Read the model definition and answer for the solid it produces. Units are mm, in the model's axes. A direction names the side the tool comes from. Coordinates: 2 decimals unless noted, no trailing zeros. Loops run counter-clockwise (first coordinate to the right, second up) from the corner with the lowest first, then second, coordinate; pieces in that order, holes last. Notation, with made-up numbers: (29.25, -32.5) -> (82.25, -32.5) arc R15 cw to (82.25, -9.5) -> close; hole circle Ø10 at (35.25, -6.75). An arc over 180 degrees is marked (long way). Answer as CSV lines item,"result".
```python
from build123d import *

# Parameters (mm, degrees)
F2_SIZE2 = 1
F2_SIZE  = 1


with BuildPart() as f1:
    # F0 (on Front) → F1 (revolve)
    with BuildSketch(Plane.XZ):
        Polygon((4, 35), (0, 35), (0, -35), (4, -35), (4, -33), (3, -33), (3, -32), (4, -32), (4, 32), (3, 32), (3, 33), (4, 33), align=None)
    revolve(axis=Axis((0, 0, 0), (0, 0, -1)))

    # F2
    f2_edges = [f1.edges().sort_by_distance(p)[0] for p in [
        (-4, 0, 35),
        (-4, 0, -35),
    ]]
    chamfer(f2_edges, length=F2_SIZE, length2=F2_SIZE2)


solid = f1.part
```
Q1. For faces 1 (the face through (-1, -3, 33)), 2 (the face through (-0.867, 3.905, 0.448)), determine the directions among +Z, -Z, +X, -X, +Y, -Y from which every point of the face is accessible in a straight line to the end or side of a thin tool.
Results:
face 1,"none"
face 2,"+Z, -Z"
Q2. Find the intervals of material crossed by probe 1 along Z at (x, y) = (-2.5, -2.75); probe 2 along Z at (x, y) = (-3, -2); probe 3 along X at (y, z) = (0.25, -10), in increasing order. Write a range as [from, to].
Results:
probe 1,"z = [-34.28, -33], [-32, 32], [33, 34.28]"
probe 2,"z = [-34.39, -33], [-32, 32], [33, 34.39]"
probe 3,"x = [-3.99, 3.99]"
Q3. A cutting plane is placed at A-A, the plane z = 1. Write down the section's boundary in (x, y), and give its area (3 significant figures).
Results:
outline,"circle Ø8 at (0, 0)"
area,"50.3 mm²"
Q4. For a pull along Z with two mould halves and no side action, classify faces 3 (the face through (1, -3, 32)), 4 (the face through (-0.867, 3.905, 33.507)), 5 (the face through (0, 0, 35)) as pulls with the +Z half, pulls with the -Z half, needs draft (parallel to the pull), parting line crosses it, or undercut.
Results:
face 3,"undercut"
face 4,"needs draft"
face 5,"pulls with the +Z half"
Q5. Given pin 1 Ø3 at (x, z) = (3, 6) entering from +Y, flat-ended and moving along its own axis, determine where the tip first touches the part or whether it passes through.
Results:
pin 1,"stops at y = 3.71"
